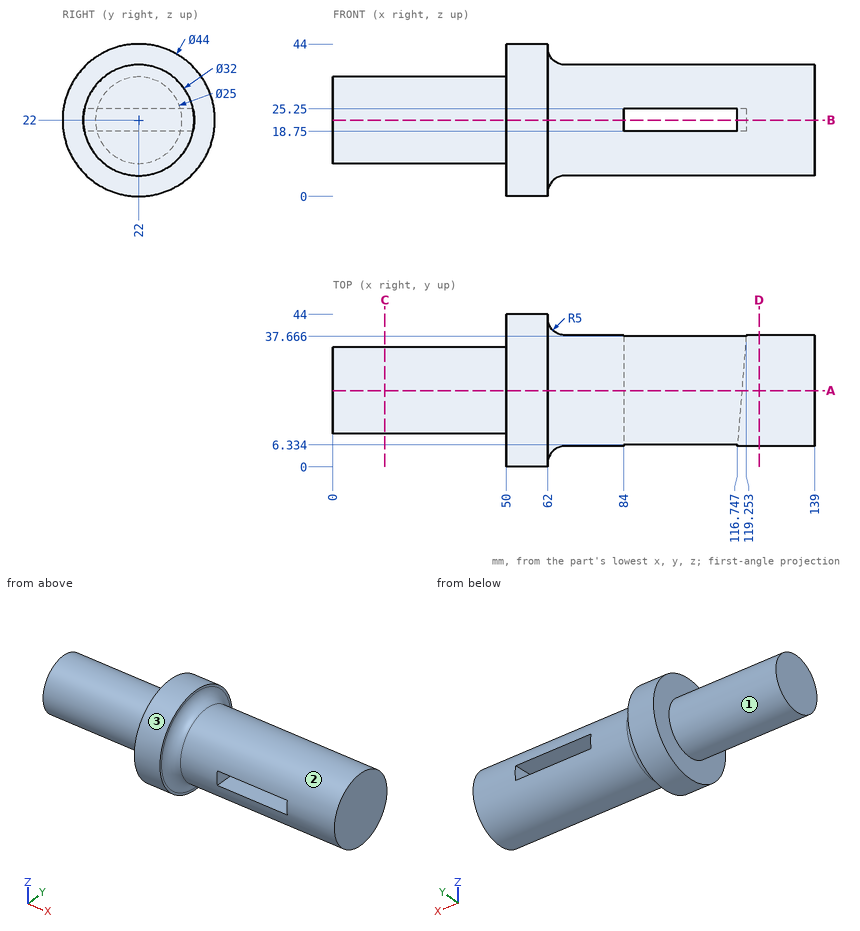
Geometry check sheet. Reference: drawing and pictorial views, mm from the part's lowest x, y, z. A direction names the side the tool comes from. Round coordinates to 2 decimals unless told otherwise and drop trailing zeros. Write each loop counter-clockwise with the first axis right and the second up, starting at its lowest first coordinate (ties: lowest second). Pieces come first, ordered by that corner, then holes.
(1) Section check B-B (z = 22). Enter the section's corners in (x, y).
Returned:
outline: (0, 9.5) - (50, 9.5) - (50, 0) - (62, 0) - (62, 1) arc R5 cw to (67, 6) - (84, 6) - (84, 38) - (67, 38) arc R5 cw to (62, 43) - (62, 44) - (50, 44) - (50, 34.5) - (0, 34.5) - close; (116.72, 6) - (139, 6) - (139, 38) - (119.28, 38) - close
(2) Material ranges on line 1 (X direction, y = 35, z = 4.5); line 2 (X direction, y = 20.5, z = 23); line 3 (Z direction, x = 111, y = 26), recorded low to high.
Returned:
line 1: x = 50 to 62
line 2: x = 0 to 84, 117.88 to 139
line 3: z = 6.51 to 18.75, 25.25 to 37.49
(3) Section check A-A (y = 22). Enter the section's corners in (x, z).
Returned:
outline: (0, 9.5) - (50, 9.5) - (50, 0) - (62, 0) - (62, 1) arc R5 cw to (67, 6) - (139, 6) - (139, 38) - (67, 38) arc R5 cw to (62, 43) - (62, 44) - (50, 44) - (50, 34.5) - (0, 34.5) - close; hole (84, 18.75) - (118, 18.75) - (118, 25.25) - (84, 25.25) - close
(4) Depth check by flat-ended pin: pin 1 Ø2 at (x, z) = (75.5, 10.5) entering from -Y; pin 2 Ø10 at (x, z) = (77, 14.5) entering from -Y; pin 3 Ø2 at (x, y) = (46, 16.5) entering from -Z. Enter the tip coordinate at first touch or a pass-through.
Returned:
pin 1: stops at y = 9.93
pin 2: stops at y = 6.2
pin 3: stops at z = 10.34
(5) Access from +Z, -Z, +X, -X, +Y, -Y to the whole of each face (thin tool, end or side, straight path). Record for the marked faces 1, 2 and 3.
Returned:
face 1: -X
face 2: +X
face 3: +X, -X
(6) Section check C-C (x = 15). Enter the section's corners in (y, z), plus the area to 3 significant figures.
Returned:
outline: circle Ø25 at (22, 22)
area: 491 mm2
(7) Section check D-D (x = 123). Enter the section's corners in (y, z), plus the area to 3 significant figures.
Returned:
outline: circle Ø32 at (22, 22)
area: 804 mm2
